Autodesk Inventor part; units mm, degrees
ref_plane "Start Plane" through (0, 0, 19.0963) normal (0, 0, 1) x (1, 0, 0)
ref_plane "End Plane" through (0, 0, 680.7758) normal (0, 0, 1) x (1, 0, 0)
ref_plane "Work Plane4" through (-9, -478.7803, -721.7447) normal (0, -0.9444582, 0.3286315) x (1, 0, 0)
ref_plane "Start Plane" through (0, 0, 19.0963) normal (0, 0, 1) x (1, 0, 0)
ref_plane "End Plane" through (0, 0, 680.7758) normal (0, 0, 1) x (1, 0, 0)
sketch "Sketch" plane through (0, 0, 0) normal (0, 0, 1) x (1, 0, 0)
  line L0 (-15, -9) -> (-15, 9)
  line L1 (-9, 15) -> (9, 15)
  line L2 (15, 9) -> (15, -9)
  line L3 (9, -15) -> (-9, -15)
  arc A0 (-15, -9) -> (-9, -15) centre (-9, -9) ccw
  arc A1 (-9, 15) -> (-15, 9) centre (-9, 9) ccw
  arc A2 (15, 9) -> (9, 15) centre (9, 9) ccw
  arc A3 (9, -15) -> (15, -9) centre (9, -9) ccw
  arc A4 (-9, 12) -> (-12, 9) centre (-9, 9) ccw
  line L4 (-9, 12) -> (9, 12)
  arc A5 (12, 9) -> (9, 12) centre (9, 9) ccw
  line L5 (12, 9) -> (12, -9)
  arc A6 (9, -12) -> (12, -9) centre (9, -9) ccw
  line L6 (9, -12) -> (-9, -12)
  arc A7 (-12, -9) -> (-9, -12) centre (-9, -9) ccw
  line L7 (-12, -9) -> (-12, 9)
  line L8 (0, 22.7397) -> (0, -22.7397) construction
  line L9 (-22.7397, 0) -> (22.7397, 0) construction
  dimension "d7" = 6
  dimension "d10" = 30
  dimension "d11" = 30
  dimension "d12" = 3
  dimension "d15" = 15
  dimension "d16" = 15
extrude "Body" add sketch "Sketch" along normal up to surface (661.6794 mm away) from surface at 19.0963
sketch "Sketch3" plane through (0, 0, 0) normal (0, 0, 1) x (1, 0, 0)
  line L0 (0, 0) -> (10, 0)
ref_plane "Work Plane3" through (0, 0, 0) normal (0, -1, 0) x (1, 0, 0)
ref_plane "Work Plane4" through (-9, -478.7803, -721.7447) normal (0, -0.9444582, 0.3286315) x (1, 0, 0)
split "Split1" plane through (-9, -478.7803, -721.7447) removes the side toward (0, -0.9444582, 0.3286315)
ref_plane "Work Plane5" through (9, -289.8887, -787.471) normal (0, 0.9444582, -0.3286315) x (1, 0, 0)
split "Split2" plane through (9, -289.8887, -787.471) removes the side toward (0, 0.9444582, -0.3286315)
ref_plane "Work Plane6" through (-9, -4.9295, 685.7053) normal (0, 0.3286315, 0.9444582) x (1, 0, 0)
split "Split3" plane through (-9, -4.9295, 685.7053) removes the side toward (0, 0.3286315, 0.9444582)
sketch "Sketch4" plane through (0, 0, 0) normal (0, -1, 0) x (1, 0, 0)
  line L0 (-2, 19.0963) -> (12, 19.0963)
  line L1 (-2, 680.7758) -> (12, 680.7758)
  dimension "d18" = 661.6794
equation "\"d7\" = G_IR"
equation "\"d10\" = G_H"
equation "\"d11\" = G_W"
equation "\"d12\" = G_T"
equation "\"d15\" = 0.5 * d10"
equation "\"d16\" = 0.5 * d11"
equation "\"d3\" = G_L"
equation "\"G_W\" = 30"
equation "\"G_H\" = 30"
equation "\"G_T\" = 3"
equation "\"G_IR\" = 6"
equation "\"G_L\" = d18"
equation "\"G_OFFSET_START\" = -19.09635"
equation "\"G_OFFSET_END\" = -19.09635"
equation "\"d13\" = -G_OFFSET_START"
equation "\"d14\" = G_OFFSET_END + B_L"
equation "\"B_L\" = 699.87213"
properties part number "DIN EN 10219-2 - 30 x 30 x 3  - 661.68" material "Steel, Mild"
Geometry check sheet. Reference: the model listing, model coordinates, mm. A direction names the side the tool comes from. Give positions to 0.01 mm unless a question says otherwise; leave off trailing zeros. Order: outer loops, then holes, each group sorted by start corner. A loop starts at its lowest first (then second) coordinate and runs counter-clockwise, first axis right, second up.
1) Material ranges on probe 1 along Y at (x, z) = (-8.25, 443); probe 2 along Y at (x, z) = (-9.75, 340), recorded low to high.
Results are:
probe 1: y = -15 to -12, 12 to 15
probe 2: y = -14.95 to -11.9, 11.9 to 14.95
2) Cross-section at C-C (y = -3). Record the boundary of the cut face in (x, z).
Results are:
outline: (-15, 37.02) - (-12, 37.02) - (-12, 645.61) - (-15, 645.61) - close; (12, 37.02) - (15, 37.02) - (15, 645.61) - (12, 645.61) - close
3) Tool access check on faces 1 (the flat face through (0, -12, 315)), 2 (the flat face through (15, 0, 345)). Record the directions out of +Z, -Z, +X, -X, +Y, -Y that give a thin tool (end or side, any length) a straight path to the whole face; none if there is none.
Results are:
face 1: +Z, -Z
face 2: +Z, -Z, +X, +Y, -Y
4) Cross-section at A-A (x = 3.75). Record the boundary of the cut face in (y, z).
Results are:
outline: (-15, 19.1) - (-12, 19.1) - (-12, 619.74) - (-15, 611.12) - close; (12, 80.13) - (15, 88.75) - (15, 678.77) - (12, 679.81) - close
5) Cross-section at B-B (z = 511). Record the boundary of the cut face in (x, y).
Results are:
outline: (-15, -9) arc R6 ccw to (-9, -15) - (9, -15) arc R6 ccw to (15, -9) - (15, 9) arc R6 ccw to (9, 15) - (-9, 15) arc R6 ccw to (-15, 9) - close; hole (-12, -9) arc R3 ccw to (-9, -12) - (9, -12) arc R3 ccw to (12, -9) - (12, 9) arc R3 ccw to (9, 12) - (-9, 12) arc R3 ccw to (-12, 9) - close
6) Draft check along Y on faces 3 (the flat face through (0, 12, 376)), 4 (the flat face through (-15, 0, 345)), 5 (the flat face through (12.15, -5.63, 638.05)), 6 (the flat face through (0, 15, 380)). Enter one of: released by +Y, released by -Y, zero draft, split by the parting line, or undercut.
Results are:
face 3: undercut
face 4: zero draft
face 5: released by -Y
face 6: released by +Y
